Read the model definition and answer for the solid it produces. Units are mm, in the model's axes. A direction names the side the tool comes from. Coordinates: 2 decimals unless noted, no trailing zeros. Order: outer loops, then holes, each group sorted by start corner. A loop starts at its lowest first (then second) coordinate and runs counter-clockwise, first axis right, second up. Notation, with made-up numbers: (9.25, 62.25) -> (27.25, 62.25) arc R35 ccw to (27.25, 98.25) -> close; hole circle Ø6 at (77, 77.25). An arc over 180 degrees is marked (long way). Use CSV: the item, a comma, the result in double quotes.
```python
from build123d import *

# Parameters (mm, degrees)
SKETCH1_R           = 81
BOSS_EXTRUDE1_DEPTH = 12
SKETCH2_R           = 76
CUT_EXTRUDE1_DEPTH  = 7
SKETCH3_R           = 32
CUT_EXTRUDE2_DEPTH  = 235.410963907
BOSS_EXTRUDE2_DEPTH = 50
SKETCH5_R           = 1.6
CUT_EXTRUDE3_DEPTH  = 6
FILLET1_R           = 4
FILLET2_R           = 2


with BuildPart() as part:
    # Sketch1 → Boss-Extrude1 (new body)
    with BuildSketch(Plane(origin=(0, 0, 0), x_dir=(1, 0, 0), z_dir=(0, 1, 0))):
        with Locations(Location((105.5, 60.5, 0), (0, 0, 270))):
            Circle(SKETCH1_R)
    extrude(amount=BOSS_EXTRUDE1_DEPTH)

    # Sketch2 → Cut-Extrude1 (cut)
    with BuildSketch(Plane.XZ):
        with Locations(Location((105.5, -60.5, 0), (0, 0, 270))):
            Circle(SKETCH2_R)
    extrude(amount=-CUT_EXTRUDE1_DEPTH, mode=Mode.SUBTRACT)

    # Sketch3 → Cut-Extrude2 (cut, through all)
    with BuildSketch(Plane(origin=(0, 12, 0), x_dir=(1, 0, 0), z_dir=(0, 1, 0))):
        with Locations(Location((105.5, 60.5, 0), (0, 0, 270))):
            Circle(SKETCH3_R)
    extrude(amount=-CUT_EXTRUDE2_DEPTH, mode=Mode.SUBTRACT)

    # Sketch4 → Boss-Extrude2 (add)
    with BuildSketch(Plane(origin=(0, 12, 0), x_dir=(1, 0, 0), z_dir=(0, 1, 0))):
        with BuildLine():
            ThreePointArc((140.957721303, 45.5), (67, 60.5), (140.957721303, 75.5))
            Line((140.957721303, 75.5), (145.775366264, 75.5))
            Line((145.775366264, 75.5), (146.331972766, 75.5))
            ThreePointArc((146.331972766, 75.5), (145.74451839, 77.011472968), (145.101136347, 78.5))
            ThreePointArc((145.101136347, 78.5), (62, 60.5), (145.101136347, 42.5))
            ThreePointArc((145.101136347, 42.5), (145.74451839, 43.988527032), (146.331972766, 45.5))
            Line((146.331972766, 45.5), (145.775366264, 45.5))
            Line((145.775366264, 45.5), (140.957721303, 45.5))
        make_face()
        with BuildLine():
            Line((146.331972766, 75.5), (145.775366264, 75.5))
            Line((145.775366264, 75.5), (145.775366264, 45.5))
            Line((145.775366264, 45.5), (146.331972766, 45.5))
            ThreePointArc((146.331972766, 45.5), (147.885391427, 50.715900981), (148.775366264, 56.084949069))
            Line((148.775366264, 56.084949069), (148.775366264, 64.915050931))
            ThreePointArc((148.775366264, 64.915050931), (147.885391427, 70.284099019), (146.331972766, 75.5))
        make_face()
        with BuildLine():
            ThreePointArc((145.101136347, 78.5), (145.74451839, 77.011472968), (146.331972766, 75.5))
            Line((146.331972766, 75.5), (148.775366264, 75.5))
            Line((148.775366264, 75.5), (148.775366264, 78.5))
            Line((148.775366264, 78.5), (145.101136347, 78.5))
        make_face()
        with BuildLine():
            Line((148.775366264, 75.5), (146.331972766, 75.5))
            ThreePointArc((146.331972766, 75.5), (147.885391427, 70.284099019), (148.775366264, 64.915050931))
            Line((148.775366264, 64.915050931), (148.775366264, 75.5))
        make_face()
        with BuildLine():
            ThreePointArc((148.775366264, 56.084949069), (147.885391427, 50.715900981), (146.331972766, 45.5))
            Line((146.331972766, 45.5), (148.775366264, 45.5))
            Line((148.775366264, 45.5), (148.775366264, 56.084949069))
        make_face()
        with BuildLine():
            Line((148.775366264, 45.5), (146.331972766, 45.5))
            ThreePointArc((146.331972766, 45.5), (145.74451839, 43.988527032), (145.101136347, 42.5))
            Line((145.101136347, 42.5), (148.775366264, 42.5))
            Line((148.775366264, 42.5), (148.775366264, 45.5))
        make_face()
    extrude(amount=BOSS_EXTRUDE2_DEPTH)

    # Sketch5 → Cut-Extrude3 (cut)
    with BuildSketch(Plane(origin=(148.775366264, 0, 0), x_dir=(0, 0, -1), z_dir=(1, 0, 0))):
        with Locations((52.5, 52)):
            Circle(SKETCH5_R)
        with Locations((68.5, 52)):
            Circle(SKETCH5_R)
        with Locations((68.5, 17)):
            Circle(SKETCH5_R)
        with Locations((52.5, 17)):
            Circle(SKETCH5_R)
    extrude(amount=-CUT_EXTRUDE3_DEPTH, mode=Mode.SUBTRACT)

    # Fillet1
    fillet1_edges = [part.edges().sort_by_distance(p)[0] for p in [
        (146.938251306, 12, -42.5),
        (145.101136347, 37, -42.5),
        (62, 12, -60.5),
        (145.101136347, 37, -78.5),
        (146.938251306, 12, -78.5),
    ]]
    fillet(fillet1_edges, radius=FILLET1_R)

    # Fillet2
    fillet2_edges = [part.edges().sort_by_distance(p)[0] for p in [
        (105.5, 7, 15.5),
    ]]
    fillet(fillet2_edges, radius=FILLET2_R)


solid = part.part
```
Item 1: Straight lines are drawn through the part: line 1 along Y through (x, z) = (147, -68.5); line 2 along Z through (x, y) = (105, 9); line 3 along X through (y, z) = (42, -60). For each, find the intervals that lie inside material, in ascending order.
Return value:
line 1,"y = 7 to 15.4, 18.6 to 50.4, 53.6 to 62"
line 2,"z = -141.5 to -92.5, -28.5 to 20.5"
line 3,"x = 62 to 67, 145.78 to 148.78"
Item 2: Each of these flat-tipped pins is pushed along its axis until it touches: P1, Ø3, axis at y = 17, z = -52.5, coming from the -X side; P2, Ø1, axis at y = 26, z = -95.5, coming from the +X side; P3, Ø4, axis at x = 144.5, y = 43.5, coming from the -Z side; P4, Ø1, axis at x = 51, z = 2.5, coming from the -Y side. Where does it stop, or does it pass through?
Return value:
P1,"stops at x = 62.49"
P2,"stops at x = 132"
P3,"stops at z = -83.37"
P4,"passes through"
Item 3: Find section A-A, the plane y = 25.5. Give the vertices of the cut face in (x, z).
Return value:
outline,"(144.05, -80.65) arc R4 cw to (147.6, -78.5) -> (148.78, -78.5) -> (148.78, -42.5) -> (147.6, -42.5) arc R4 cw to (144.05, -40.35) arc R43.5 ccw (long way) to start; hole (140.96, -75.5) -> (145.78, -75.5) -> (145.78, -45.5) -> (140.96, -45.5) arc R38.5 ccw (long way) to start"
Item 4: A tool of negligible diameter and unlimited length cuts with its end or side. For faces 1 (the cylindrical face through (148.195, 13.141, -41.297)), 2 (the cylindrical face through (148.178, 13.141, -79.703)), 3 (the flat face through (148.775, 37, -60)), 4 (the flat face through (90, 7, -92)), 5 (the cylindrical face through (62.03, 38.68, -62.12)), from which of +Z, -Z, +X, -X, +Y, -Y can it reach the whole face along a straight path? Write none if from no direction.
Return value:
face 1,"+Z, +X, +Y"
face 2,"-Z, +X, +Y"
face 3,"+Z, -Z, +X, +Y"
face 4,"-Y"
face 5,"+Y"
